Work out the finished part from the listing and answer in its coordinate system (mm). Face numbers are marked on the shaded views. Round coordinates to 2 decimals unless told otherwise and drop trailing zeros. Write each loop counter-clockwise with the first axis right and the second up, starting at its lowest first coordinate (ties: lowest second). Pieces come first, ordered by that corner, then holes.
1. Straight lines are drawn through the part: probe 1 along Z at (x, y) = (12, 61); probe 2 along Z at (x, y) = (25, 47.5); probe 3 along Y at (x, z) = (33, -23). For each, find the intervals that lie inside material, in ascending order.
2. Find section C-C (z = -12). Write down the section's boundary in (x, y).
3. Find section D-D (x = 51.5). Write down the section's boundary in (y, z).
4. Find section A-A (y = 53). Write down the section's boundary in (x, z).
5. Find section B-B (x = 18.5). Write down the section's boundary in (y, z).
6. Determine the mould class of the marked faces 1, 2 and 3 for opening direction Z: pulls with the +Z half, pulls with the -Z half, needs draft (parallel to the pull), parting line crosses it, or undercut.
```python
from build123d import *

# Parameters (mm, degrees)
SKETCH3_W           = 60.452
SKETCH3_H           = 88.9
BOSS_EXTRUDE1_DEPTH = 63.5
CUT_EXTRUDE1_DEPTH  = 63.5
BOSS_EXTRUDE2_DEPTH = 63.5


with BuildPart() as part:
    # Sketch3 → Boss-Extrude1 (new body)
    with BuildSketch(Plane(origin=(0, 0, 0), x_dir=(1, 0, 0), z_dir=(0, 1, 0))):
        with Locations((30.226, 44.45)):
            Rectangle(SKETCH3_W, SKETCH3_H)
    extrude(amount=BOSS_EXTRUDE1_DEPTH)

    # Sketch4 → Cut-Extrude1 (cut)
    with BuildSketch(Plane(origin=(0, 0, 0), x_dir=(0, 0, -1), z_dir=(1, 0, 0))):
        Polygon((0, 16.002), (88.9, 41.402), (88.9, 63.5), (0, 63.5), align=None)
    extrude(amount=CUT_EXTRUDE1_DEPTH, mode=Mode.SUBTRACT)

    # Sketch5 → Boss-Extrude2 (add)
    with BuildSketch(Plane(origin=(0, 0, 0), x_dir=(1, 0, 0), z_dir=(0, 1, 0))):
        Polygon((33.110714286, 57.15), (44.45, 88.9), (18.107802509, 88.9), (0, 88.9), (0, 57.15), align=None)
        Polygon((12.7, 0), (24.039285714, 31.75), (0, 31.75), (0, 0), align=None)
    extrude(amount=BOSS_EXTRUDE2_DEPTH)


solid = part.part
```
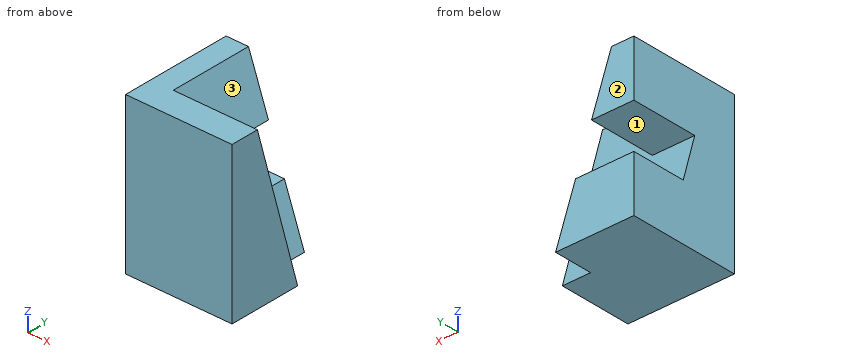
Worked answers:
1. probe 1: z = -88.9 to -57.15, -31.75 to 0
1. probe 2: z = -88.9 to -57.15
1. probe 3: y = 0 to 22.57
2. outline: (0, 0) - (60.45, 0) - (60.45, 19.43) - (16.99, 19.43) - (16.99, 63.5) - (0, 63.5) - close
3. outline: (0, -88.9) - (41.4, -88.9) - (16, 0) - (0, 0) - close
4. outline: (0, -88.9) - (44.45, -88.9) - (33.11, -57.15) - (0, -57.15) - close; (0, -31.75) - (24.04, -31.75) - (12.7, 0) - (0, 0) - close
5. outline: (0, -88.9) - (63.5, -88.9) - (63.5, -57.15) - (32.33, -57.15) - (25.07, -31.75) - (63.5, -31.75) - (63.5, -16.24) - (20.64, -16.24) - (16, 0) - (0, 0) - close
6. face 1: undercut
6. face 2: needs draft
6. face 3: pulls with the +Z half
